Here's how the part is built. I have some questions about the finished solid (model axes, mm). Face numbers are marked on the shaded views. A direction names the side the tool comes from. Give positions to 0.01 mm unless a question says otherwise; leave off trailing zeros. Write each loop counter-clockwise with the first axis right and the second up, starting at its lowest first coordinate (ties: lowest second). Pieces come first, ordered by that corner, then holes. Notation, with made-up numbers: (41.5, 54.25) -> (61.5, 54.25) arc R16 cw to (61.5, 71.25) -> close; hole circle Ø6 at (83.25, 27). An arc over 180 degrees is marked (long way). Use one line per item in the form item = value.
Autodesk Fusion 360 part; units mm, degrees
sketch "Sketch1" plane through (0, 0, 0) normal (0, 0, 1) x (1, 0, 0)
  line L0 (21, 14.5) -> (-21, 14.5)
  line L1 (-21, 14.5) -> (-21, -14.5)
  line L2 (-21, -14.5) -> (21, -14.5)
  line L3 (21, -14.5) -> (21, 14.5)
  line L4 (21, 14.5) -> (-21, -14.5) construction
  line L5 (-21, 14.5) -> (21, -14.5) construction
  dimension "d1" = 42
  dimension "d2" = 29
extrude "Extrude1" add sketch "Sketch1" along normal blind 15
fillet "Fillet1" radius 8 2 edges at (21, -14.5, 7.5) (21, 14.5, 7.5)
sketch "Sketch2" plane through (0, 0, 0) normal (0, 0, -1) x (1, 0, 0)
  arc A0 (13, -14.5) -> (21, -6.5) centre (13, -6.5) ccw
  line L0 (21, -6.5) -> (21, 6.5)
  arc A1 (21, 6.5) -> (13, 14.5) centre (13, 6.5) ccw
  line L1 (13, 14.5) -> (-21, 14.5)
  line L2 (-21, 14.5) -> (-21, -14.5)
  line L3 (-21, -14.5) -> (13, -14.5)
  line L4 (-21, -14.5) -> (-11, -14.5)
  line L5 (-11, -14.5) -> (-11, -4.5)
  line L6 (-11, -4.5) -> (-21, -4.5)
  line L7 (-21, -4.5) -> (-21, -14.5)
  dimension "d6" = 10
  dimension "d7" = 10
extrude "Extrude2" add sketch "Sketch2" along normal blind 9 contours L2 L3 L4 L5 L6 L7
sketch "Sketch3" plane through (0, 0, 0) normal (0, 0, -1) x (1, 0, 0)
  line L0 (-11, -4.5) -> (-11, -14.5)
  line L1 (-11, -14.5) -> (13, -14.5)
  arc A0 (13, -14.5) -> (21, -6.5) centre (13, -6.5) ccw
  line L2 (21, -6.5) -> (21, 6.5)
  arc A1 (21, 6.5) -> (13, 14.5) centre (13, 6.5) ccw
  line L3 (13, 14.5) -> (-21, 14.5)
  line L4 (-21, 14.5) -> (-21, -4.5)
  line L5 (-21, -4.5) -> (-11, -4.5)
  line L6 (-14.2092, -3.0986) -> (16.0935, -3.0986) construction
  line L7 (16.0935, -3.0986) -> (16.0935, 6.9014) construction
  line L8 (16.0935, 6.9014) -> (-14.2092, 6.9014) construction
  line L9 (-14.2092, 6.9014) -> (-14.2092, -3.0986) construction
sketch "Sketch4" plane through (0, 0, 15) normal (0, 0, 1) x (-1, 0, 0)
  arc A0 (-21, -6.5) -> (-13, -14.5) centre (-13, -6.5) ccw
  line L0 (-13, -14.5) -> (21, -14.5)
  line L1 (21, -14.5) -> (21, 14.5)
  line L2 (21, 14.5) -> (-13, 14.5)
  arc A1 (-13, 14.5) -> (-21, 6.5) centre (-13, 6.5) ccw
  line L3 (-21, 6.5) -> (-21, -6.5)
  line L4 (-13, 14.5) -> (-29, 14.5)
  line L5 (-29, 14.5) -> (-29, -20)
  line L6 (-29, -20) -> (-13, -20)
  line L7 (-13, -20) -> (-13, 14.5)
extrude "Extrude3" cut sketch "Sketch4" against normal blind 13.4 contours A0 A1 L3 L7 | A0 A1 L3 L4 L5 L6 L7
equation "d10 = -15 mm + 1.6 mm"
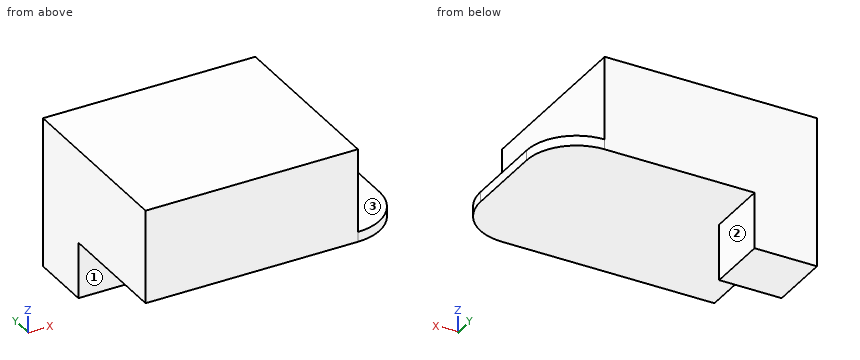
Q1. I want a section at D-D, the plane y = -2.75. Write out the boundary of the cut face in (x, z), and give its area (3 significant figures).
Result set:
outline = (-21, 0) -> (21, 0) -> (21, 1.6) -> (13, 1.6) -> (13, 15) -> (-21, 15) -> close
area = 523 mm2
Q2. Will these pins go through, and if not, where does the flat tip stop? pin 1 Ø3 at (x, y) = (15, 2) entering from -Z; pin 2 Ø4.5 at (x, z) = (-17.5, -2.5) entering from -Y; pin 3 Ø2.5 at (y, z) = (8.5, -4.5) entering from +X; pin 4 Ø4 at (y, z) = (-4, -2.5) entering from +X.
Result set:
pin_1 = 0
pin_2 = 4.5
pin_3 = -11
pin_4 = through
Q3. I want a section at C-C, the plane z = -5.5. Write out the boundary of the cut face in (x, y), and give its area (3 significant figures).
Result set:
outline = (-21, 4.5) -> (-11, 4.5) -> (-11, 14.5) -> (-21, 14.5) -> close
area = 100 mm2
Q4. If I drill on line 1 along X through (y, z) = (-1.25, 4.5); line 2 along Z through (x, y) = (3, -9); line 3 along X through (y, z) = (13.5, -5.5), over which ranges is the centre line in solid material (lowest first)? Write a range as from..to.
Result set:
line_1 = -21..13
line_2 = 0..15
line_3 = -21..-11
Q5. I want a section at A-A, the plane y = 9.5. Write out the boundary of the cut face in (x, z), and give its area (3 significant figures).
Result set:
outline = (-21, -9) -> (-11, -9) -> (-11, 0) -> (20.42, 0) -> (20.42, 1.6) -> (13, 1.6) -> (13, 15) -> (-21, 15) -> close
area = 612 mm2
Q6. I want a section at B-B, the plane x = -16.5. Write out the boundary of the cut face in (y, z), and give its area (3 significant figures).
Result set:
outline = (-14.5, 0) -> (4.5, 0) -> (4.5, -9) -> (14.5, -9) -> (14.5, 15) -> (-14.5, 15) -> close
area = 525 mm2
Q7. Which directions (+Z, -Z, +X, -X, +Y, -Y) give clear straight access to the entire face, cutting with the end or side of a thin tool? Please do the marked faces 1, 2 and 3.
Result set:
face_1 = -Z, +X, -X, -Y
face_2 = -Z, +X, +Y, -Y
face_3 = +Z, +X, +Y, -Y
